Design review of the part built by this model. Coordinates are the model's own, in mm. A direction names the side the tool comes from. Coordinates: 2 decimals unless noted, no trailing zeros. Write each loop counter-clockwise with the first axis right and the second up, starting at its lowest first coordinate (ties: lowest second). Pieces come first, ordered by that corner, then holes. Notation, with made-up numbers: (-2.5, 62) - (16.5, 62) arc R19 ccw to (16.5, 89) - close; hole circle Ø8 at (67.5, 26.25). An arc over 180 degrees is marked (long way). Answer as CSV lines item,"result". Start each with the question number.
Q1. Mouldability with a two-part tool opening along X and no side actions: class faces 3 (the face through (113, -28, 83)), 4 (the face through (0.966, 1.09, -34.521)), 5 (the face through (-2, -27.7, 141)) as pulls with the +X half, pulls with the -X half, needs draft (parallel to the pull), parting line crosses it, or undercut.
Q2. We need section D-D (y = -14). Write out the cut boundary in (x, z).
Q3. Clearance check with flat-ended pins moving along their axes: pin 1 (2 mm diameter, centred on x = 42.5, y = -23.5, fed in from -Z); pin 2 (11.5 mm diameter, centred on x = 74, z = 50, fed in from -Y); pin 3 (3 mm diameter, centred on x = -48.5, z = 155.5, fed in from +Y). State where each tip first meets the part, or that it passes through.
Q4. We need section B-B (x = 74). Write out the cut boundary in (y, z).
Q5. We need section A-A (z = 50). Write out the cut boundary in (x, y), plus the area to 3 significant figures.
Q6. Machinability: for faces 1 (the face through (108, 1, -57)), 2 (the face through (2, 0, -2)), which of the approach directions +Z, -Z, +X, -X, +Y, -Y give a long, thin tool a straight path to every point of the face, cutting with its end or side? Answer none if there is none.
Q7. For line 1 along Z through (x, y) = (25, -23); line 2 along X through (y, z) = (-28, 81); line 3 along Y through (x, z) = (-65, 142), list the stretches that pass through material, from the lowest coordinate up. Write a range as [from, to].
Q8. We need section C-C (x = -3). Write out the cut boundary in (y, z).
from build123d import *

# Parameters (mm, degrees)
SKETCH1_W                    = 2.15
SKETCH1_H                    = 124
BASE_FLANGE1_DEPTH           = 113
CHAMFER1_SIZE                = 10
EDGE_FLANGE1_STRIP_W         = 14.6
EDGE_FLANGE1_STRIP_H         = 2.15
EDGE_FLANGE1_STRIP_CUT_DEPTH = 226
EDGE_FLANGE1_DEPTH           = 226
EDGE_FLANGE2_STRIP_W         = 14.6
EDGE_FLANGE2_STRIP_H         = 2.15
EDGE_FLANGE2_STRIP_CUT_DEPTH = 226
EDGE_FLANGE2_DEPTH           = 226
EDGE_FLANGE3_STRIP_W         = 14.6
EDGE_FLANGE3_STRIP_H         = 2.15
EDGE_FLANGE3_STRIP_CUT_DEPTH = 226
EDGE_FLANGE3_DEPTH           = 226
SKETCH15_R                   = 11
CUT_EXTRUDE1_DEPTH           = 250.252928769
SKETCH16_R                   = 4
CUT_EXTRUDE2_DEPTH           = 250.252928769
LPATTERN1_COUNT              = 7
LPATTERN1_PITCH              = 20
SKETCH17_R                   = 5
CUT_EXTRUDE3_DEPTH           = 250.252928769


# Sheet-metal steps are written as plain solids
with BuildPart() as part:
    # Sketch1 → Base-Flange1 (new, symmetric)
    with BuildSketch(Plane(origin=(0, 0, 0), x_dir=(0, -1, 0), z_dir=(1, 0, 0))):
        with Locations((-1.075, 0)):
            Rectangle(SKETCH1_W, SKETCH1_H)
    extrude(amount=BASE_FLANGE1_DEPTH, both=True)

    # Chamfer1
    chamfer1_edges = [part.edges().sort_by_distance(p)[0] for p in [
        (113, 1.075, -62),
        (-113, 1.075, -62),
    ]]
    chamfer(chamfer1_edges, length=CHAMFER1_SIZE)

    # Edge-Flange1 strip (across the edge) → Edge-Flange1 strip cut (cut)
    with BuildSketch(Plane(origin=(113, 0, 62), x_dir=(0, 0, -1), z_dir=(-1, 0, 0))):
        with Locations((-2.15, -1.075)):
            Rectangle(EDGE_FLANGE1_STRIP_W, EDGE_FLANGE1_STRIP_H)
    extrude(amount=EDGE_FLANGE1_STRIP_CUT_DEPTH, mode=Mode.SUBTRACT)

    # Edge-Flange1 section (across the edge) → Edge-Flange1 (add)
    with BuildSketch(Plane(origin=(113, 0, 62), x_dir=(0, 0, -1), z_dir=(-1, 0, 0))):
        with BuildLine():
            Line((0, 3), (0, 29.85))
            Line((0, 29.85), (2.15, 29.85))
            Line((2.15, 29.85), (2.15, 3))
            ThreePointArc((2.15, 3), (3.028679656, 0.878679656), (5.15, 0))
            Line((5.15, 0), (5.15, -2.15))
            ThreePointArc((5.15, -2.15), (1.508400077, -0.641599923), (0, 3))
        make_face()
    extrude(amount=EDGE_FLANGE1_DEPTH)

    # Edge-Flange2 strip (across the edge) → Edge-Flange2 strip cut (cut)
    with BuildSketch(Plane(origin=(-113, -29.85, 62), x_dir=(0, 1, 0), z_dir=(1, 0, 0))):
        with Locations((-2.15, -1.075)):
            Rectangle(EDGE_FLANGE2_STRIP_W, EDGE_FLANGE2_STRIP_H)
    extrude(amount=EDGE_FLANGE2_STRIP_CUT_DEPTH, mode=Mode.SUBTRACT)

    # Edge-Flange2 section (across the edge) → Edge-Flange2 (add)
    with BuildSketch(Plane(origin=(-113, -29.85, 62), x_dir=(0, 1, 0), z_dir=(1, 0, 0))):
        with BuildLine():
            Line((0, 3), (0, 157.85))
            Line((0, 157.85), (2.15, 157.85))
            Line((2.15, 157.85), (2.15, 3))
            ThreePointArc((2.15, 3), (3.028679656, 0.878679656), (5.15, 0))
            Line((5.15, 0), (5.15, -2.15))
            ThreePointArc((5.15, -2.15), (1.508400077, -0.641599923), (0, 3))
        make_face()
    extrude(amount=EDGE_FLANGE2_DEPTH)

    # Edge-Flange3 strip (across the edge) → Edge-Flange3 strip cut (cut)
    with BuildSketch(Plane(origin=(-113, -27.7, 219.85), x_dir=(0, 0, -1), z_dir=(1, 0, 0))):
        with Locations((-2.15, -1.075)):
            Rectangle(EDGE_FLANGE3_STRIP_W, EDGE_FLANGE3_STRIP_H)
    extrude(amount=EDGE_FLANGE3_STRIP_CUT_DEPTH, mode=Mode.SUBTRACT)

    # Edge-Flange3 section (across the edge) → Edge-Flange3 (add)
    with BuildSketch(Plane(origin=(-113, -27.7, 219.85), x_dir=(0, 0, -1), z_dir=(1, 0, 0))):
        with BuildLine():
            Line((0, 3), (0, 4.85))
            Line((0, 4.85), (2.15, 4.85))
            Line((2.15, 4.85), (2.15, 3))
            ThreePointArc((2.15, 3), (3.028679656, 0.878679656), (5.15, 0))
            Line((5.15, 0), (5.15, -2.15))
            ThreePointArc((5.15, -2.15), (1.508400077, -0.641599923), (0, 3))
        make_face()
    extrude(amount=EDGE_FLANGE3_DEPTH)

    # Sketch15 → Cut-Extrude1 (cut, through all)
    with BuildSketch(Plane.XZ.offset(29.85)):
        with Locations(Location((-64, 81.85, 0), (0, 0, 270))):
            Circle(SKETCH15_R)
    extrude(amount=-CUT_EXTRUDE1_DEPTH, mode=Mode.SUBTRACT)

    # Sketch16 → Cut-Extrude2 (cut, through all)
    with BuildSketch(Plane(origin=(0, 2.15, 0), x_dir=(1, 0, 0), z_dir=(0, 1, 0))):
        with Locations(Location((-63, 34, 0), (0, 0, 270))):
            Circle(SKETCH16_R)
    cut_extrude2 = extrude(amount=-CUT_EXTRUDE2_DEPTH, mode=Mode.SUBTRACT)

    # LPattern1: Cut-Extrude2 ×7
    with Locations(*[(i * LPATTERN1_PITCH, 0, 0) for i in range(1, LPATTERN1_COUNT)]):
        add(cut_extrude2, mode=Mode.SUBTRACT)

    # Sketch17 → Cut-Extrude3 (cut, through all)
    with BuildSketch(Plane(origin=(0, 2.15, 0), x_dir=(1, 0, 0), z_dir=(0, 1, 0))):
        with Locations(Location((74, -50, 0), (0, 0, 270))):
            Circle(SKETCH17_R)
    extrude(amount=-CUT_EXTRUDE3_DEPTH, mode=Mode.SUBTRACT)


solid = part.part
Results list:
1,face 3,"pulls with the +X half"
1,face 4,"undercut"
1,face 5,"needs draft"
2,outline,"(-113, 59.85) - (113, 59.85) - (113, 62) - (-113, 62) - close"
3,pin 1,"stops at z = 59.85"
3,pin 2,"stops at y = 0"
3,pin 3,"stops at y = -27.7"
4,outline,"(-29.85, 65) arc R5.15 ccw to (-24.7, 59.85) - (-3, 59.85) arc R3 cw to (0, 56.85) - (0, 55) - (2.15, 55) - (2.15, 56.85) arc R5.15 ccw to (-3, 62) - (-24.7, 62) arc R3 cw to (-27.7, 65) - (-27.7, 214.7) arc R3 cw to (-24.7, 217.7) - (-22.85, 217.7) - (-22.85, 219.85) - (-24.7, 219.85) arc R5.15 ccw to (-29.85, 214.7) - close; (0, -62) - (2.15, -62) - (2.15, 45) - (0, 45) - close"
5,outline,"(-113, 0) - (69, 0) - (69, 2.15) - (-113, 2.15) - close; (79, 0) - (113, 0) - (113, 2.15) - (79, 2.15) - close"
5,area,"464 mm2"
6,face 1,"-Z, +X, +Y, -Y"
6,face 2,"-Z, +X, -X, -Y"
7,line 1,"z = [59.85, 62], [217.7, 219.85]"
7,line 2,"x = [-113, -74.97], [-53.03, 113]"
7,line 3,"y = [-29.85, -27.7]"
8,outline,"(-29.85, 65) arc R5.15 ccw to (-24.7, 59.85) - (-3, 59.85) arc R3 cw to (0, 56.85) - (0, -30) - (2.15, -30) - (2.15, 56.85) arc R5.15 ccw to (-3, 62) - (-24.7, 62) arc R3 cw to (-27.7, 65) - (-27.7, 214.7) arc R3 cw to (-24.7, 217.7) - (-22.85, 217.7) - (-22.85, 219.85) - (-24.7, 219.85) arc R5.15 ccw to (-29.85, 214.7) - close; (0, -62) - (2.15, -62) - (2.15, -38) - (0, -38) - close"
